```python
from build123d import *

# Parameters (mm, degrees)
F0_R          = 2.5
F1_DEPTH      = 20
F3_DEPTH      = 25
F5_DEPTH      = 33.15069
F5_DEPTH_BACK = 22.85131


with BuildPart() as f1:
    # F0 (on Top) → F1 (new body)
    with BuildSketch(Plane.XY):
        with BuildLine():
            Line((29.14969, 36.637019), (-18.85031, 36.637019))
            ThreePointArc((-18.85031, 36.637019), (-21.678737, 35.465446), (-22.85031, 32.637019))
            Line((-22.85031, 32.637019), (-22.85031, -37.362981))
            ThreePointArc((-22.85031, -37.362981), (-21.678737, -40.191408), (-18.85031, -41.362981))
            Line((-18.85031, -41.362981), (29.14969, -41.362981))
            ThreePointArc((29.14969, -41.362981), (31.978117, -40.191408), (33.14969, -37.362981))
            Line((33.14969, -37.362981), (33.14969, 32.637019))
            ThreePointArc((33.14969, 32.637019), (31.978117, 35.465446), (29.14969, 36.637019))
        make_face()
        with Locations((-15.35031, -34.862981)):
            Circle(F0_R, mode=Mode.SUBTRACT)
        with Locations((-15.35031, -25.337981)):
            Circle(F0_R, mode=Mode.SUBTRACT)
        with Locations((25.64969, -34.862981)):
            Circle(F0_R, mode=Mode.SUBTRACT)
        with Locations((25.64969, -25.337981)):
            Circle(F0_R, mode=Mode.SUBTRACT)
        with Locations((-15.35031, 28.637019)):
            Circle(F0_R, mode=Mode.SUBTRACT)
        with Locations((25.64969, 28.637019)):
            Circle(F0_R, mode=Mode.SUBTRACT)
    extrude(amount=F1_DEPTH)

    # F2 (on face) → F3 (cut)
    with BuildSketch(Plane.XY.offset(20)):
        Polygon((5.14969, -9.362981), (-8.85031, -34.362981), (19.14969, -34.362981), align=None)
    extrude(amount=-F3_DEPTH, mode=Mode.SUBTRACT)

    # F4 (on Right) → F5 (cut, two sides)
    with BuildSketch(Plane.YZ) as f5_sk:
        Polygon((36.637019, 2), (36.637019, 20), (-41.362981, 20), (-41.362981, 10), align=None)
    extrude(amount=F5_DEPTH, mode=Mode.SUBTRACT)
    extrude(f5_sk.sketch, amount=-F5_DEPTH_BACK, mode=Mode.SUBTRACT)


solid = f1.part
```
CAD build for the part. Positions are in the model's coordinates, mm. A direction names the side the tool comes from. Coordinates: 2 decimals unless noted, no trailing zeros. Loops run counter-clockwise (first coordinate to the right, second up) from the corner with the lowest first, then second, coordinate; pieces in that order, holes last. Notation, with made-up numbers: (75.25, -27) - (83.25, -27) arc R23 ccw to (83.25, 9) - close; hole circle Ø3 at (-32, 14.5). An arc over 180 degrees is marked (long way). Return JSON: item names as keys, results as strings.
1. Probe L1, parallel to X at y = 27, z = 2.5; L2, parallel to X at y = -33.5, z = 4; L3, parallel to X at y = -10.5, z = 4.75. List the from-to ranges inside material, lowest first. Write a range as from..to.
Result:
{"L1": "x = -22.85..-17.24, -13.46..23.76, 27.54..33.15", "L2": "x = -22.85..-17.45, -13.25..-8.37, 18.67..23.55, 27.75..33.15", "L3": "x = -22.85..4.51, 5.79..33.15"}
2. Band-saw the part on B-B (z = 1). Give the cut face in (x, y), and give its area (3 significant figures).
Result:
{"outline": "(-22.85, -37.36) arc R4 ccw to (-18.85, -41.36) - (29.15, -41.36) arc R4 ccw to (33.15, -37.36) - (33.15, 32.64) arc R4 ccw to (29.15, 36.64) - (-18.85, 36.64) arc R4 ccw to (-22.85, 32.64) - close; hole circle Ø5 at (-15.35, -34.86); hole circle Ø5 at (-15.35, -25.34); hole circle Ø5 at (-15.35, 28.64); hole (-8.85, -34.36) - (19.15, -34.36) - (5.15, -9.36) - close; hole circle Ø5 at (25.65, -34.86); hole circle Ø5 at (25.65, -25.34); hole circle Ø5 at (25.65, 28.64)", "area": "3,890 mm2"}
3. Mould opens along X. For faces 3 (the cylindrical face through (32.009, 35.434, 1.188)), 4 (the flat face through (5, -41.363, 5)), 5 (the cylindrical face through (-15.9, 26.2, 1.5)) say: released by +X, released by -X, zero draft, split by the parting line, or undercut.
Result:
{"face 3": "released by +X", "face 4": "zero draft", "face 5": "undercut"}
4. 3-axis set-ups, long thin cutter, end or side, ignore diameter. For faces 1 (the flat face through (5.542, -2.909, 6.056)), 2 (the flat face through (12.25, -22.04, 3.67)): which of +Z, -Z, +X, -X, +Y, -Y reach the whole face in a straight line?
Result:
{"face 1": "+Z, +X, -X, +Y", "face 2": "+Z, -Z"}
5. Band-saw the part on A-A (x = 10). Give the cut face in (y, z), and give its area (3 significant figures).
Result:
{"outline": "(-41.36, 0) - (-34.36, 0) - (-34.36, 9.28) - (-41.36, 10) - close; (-18.02, 0) - (36.64, 0) - (36.64, 2) - (-18.02, 7.61) - close", "area": "330 mm2"}
6. Drop flat-ended pins along their axis: pin 1 (6.5 mm diameter, centred on x = 25.65, y = -25.34, fed in from +Z); pin 2 (4 mm diameter, centred on x = -13.5, y = -24.5, fed in from +Z); pin 3 (3 mm diameter, centred on x = -15.35, y = -25.34, fed in from -Z); pin 4 (8 mm diameter, centred on x = -15.35, y = 28.64, fed in from +Z). Give the stop position or say it passes through.
Result:
{"pin 1": "stops at z = 8.69", "pin 2": "stops at z = 8.47", "pin 3": "passes through", "pin 4": "stops at z = 3.23"}
7. Band-saw the part on D-D (x = 26). Give the cut face in (y, z), and give its area (3 significant figures).
Result:
{"outline": "(-41.36, 0) - (-37.34, 0) - (-37.34, 9.59) - (-41.36, 10) - close; (-32.39, 0) - (-27.81, 0) - (-27.81, 8.61) - (-32.39, 9.08) - close; (-22.86, 0) - (26.16, 0) - (26.16, 3.07) - (-22.86, 8.1) - close; (31.11, 0) - (36.64, 0) - (36.64, 2) - (31.11, 2.57) - close", "area": "366 mm2"}
8. Band-saw the part on C-C (y = -20). Give the cut face in (x, z), and give its area (3 significant figures).
Result:
{"outline": "(-22.85, 0) - (-0.81, 0) - (-0.81, 7.81) - (-22.85, 7.81) - close; (11.11, 0) - (33.15, 0) - (33.15, 7.81) - (11.11, 7.81) - close", "area": "344 mm2"}
